from build123d import *

# Parameters (mm, degrees)
F0_W     = 30
F0_H     = 30
F1_DEPTH = 2
F3_DEPTH = 15
F4_W     = 8.5
F4_H     = 8.5
F5_DEPTH = 25
F6_W     = 2
F6_H     = 8
F7_DEPTH = 15
F8_W     = 5
F8_H     = 8
F9_DEPTH = 1


with BuildPart() as f1:
    # F0 (on Front) → F1 (new body)
    with BuildSketch(Plane.XZ):
        Rectangle(F0_W, F0_H)
    extrude(amount=F1_DEPTH)

    # F2 (on face) → F3 (join)
    with BuildSketch(Plane.XZ.offset(2)):
        Polygon((5.9, -11), (5.9, -13), (11.9, -13), (11.9, 0), (5.9, 0), (5.9, -2), (9.9, -2), (9.9, -11), align=None)
        Polygon((-9.9, -2), (-5.9, -2), (-5.9, 0), (-11.9, 0), (-11.9, -13), (-5.9, -13), (-5.9, -11), (-9.9, -11), align=None)
    extrude(amount=F3_DEPTH)

    # F4 (on face) → F5 (cut)
    with BuildSketch(Plane.XZ.offset(2)):
        with Locations((0, -1.25)):
            Rectangle(F4_W, F4_H)
    extrude(amount=-F5_DEPTH, mode=Mode.SUBTRACT)

    # F6 (on face) → F7 (join)
    with BuildSketch(Plane.XZ.offset(2)):
        with Locations((-7.263201, 9)):
            Rectangle(F6_W, F6_H)
        with Locations((7.263201, 9)):
            Rectangle(F6_W, F6_H)
    extrude(amount=F7_DEPTH)

    # F8 (on face) → F9 (cut)
    with BuildSketch(Plane.XZ.offset(2)):
        with Locations((0, 7)):
            Rectangle(F8_W, F8_H)
    extrude(amount=-F9_DEPTH, mode=Mode.SUBTRACT)


solid = f1.part
For this review, take the finished solid that the model builds, in its own axes (mm). A direction names the side the tool comes from. Round coordinates to 2 decimals unless told otherwise and drop trailing zeros. Order: outer loops, then holes, each group sorted by start corner. A loop starts at its lowest first (then second) coordinate and runs counter-clockwise, first axis right, second up. Notation, with made-up numbers: (43, 50.25) -> (78, 50.25) arc R20 cw to (78, 74.25) -> close; hole circle Ø1 at (38, -9). An arc over 180 degrees is marked (long way). Write item = value, one per line. Start each with the question number.
1) Tool access review of faces 1 (the face through (7, -9, 5)), 2 (the face through (8, -9, -2)), 3 (the face through (-5.9, -9, -1)), 4 (the face through (4.25, -1, -1)): name each direction out of +Z, -Z, +X, -X, +Y, -Y from which nothing blocks a thin tool from reaching the whole face with its end or side.
2) Take a section at C-C on y = -1.5. State the section outline as (x, z) points, plus the area to 3 significant figures.
3) The part is to be moulded in two halves that separate along Z. For faces 5 (the face through (9, -9, -13)), 6 (the face through (2.5, -1.5, 6.9)), 7 (the face through (-7, -17, 9)), say which applies: +Z half, -Z half, draft (parallel to the pull), parting line (faces both ways), or undercut.
4) Take a section at B-B on x = 2. State the section outline as (y, z) points.
5) Take a section at D-D on z = -7.75. State the section outline as (x, y) points.
6) Insertion check: pin 1 (1.2 mm diameter, centred on x = 7.5, y = -8, fed in from +Z); pin 2 (8 mm diameter, centred on y = -13.5, z = 8, fed in from +X); pin 3 (1.5 mm diameter, centred on y = -4.5, z = -2, fed in from +X). Each pin has a flat end and moves straight along its axis. Give the tip position at first contact, or say it passes through.
7) Take a section at A-A on y = -10.75. State the section outline as (x, z) points, plus the area to 3 significant figures.
8) To check wall thickness, follow line 1 (Z direction, x = -8, y = -5.25); line 2 (X direction, y = -11.75, z = -5.5); line 3 (Z direction, x = -8.75, y = -11.75). State the ranges of each line that lie inside material, in increasing order. Write a range as from..to.
Verdict:
q1.face_1 = +X, -X, -Y
q1.face_2 = -Y
q1.face_3 = +Z, -Z, -Y
q1.face_4 = +Y, -Y
q2.outline = (-15, -15) -> (15, -15) -> (15, 15) -> (-15, 15) -> close; hole (-4.25, -5.5) -> (4.25, -5.5) -> (4.25, 3) -> (2.5, 3) -> (2.5, 11) -> (-2.5, 11) -> (-2.5, 3) -> (-4.25, 3) -> close
q2.area = 788 mm2
q3.face_5 = -Z half
q3.face_6 = undercut
q3.face_7 = draft
q4.outline = (-2, -15) -> (0, -15) -> (0, -5.5) -> (-2, -5.5) -> close; (-2, 11) -> (-1, 11) -> (-1, 3) -> (0, 3) -> (0, 15) -> (-2, 15) -> close
q5.outline = (-15, -2) -> (-11.9, -2) -> (-11.9, -17) -> (-9.9, -17) -> (-9.9, -2) -> (9.9, -2) -> (9.9, -17) -> (11.9, -17) -> (11.9, -2) -> (15, -2) -> (15, 0) -> (-15, 0) -> close
q6.pin_1 = 13
q6.pin_2 = 8.26
q6.pin_3 = 11.9
q7.outline = (-11.9, -13) -> (-5.9, -13) -> (-5.9, -11) -> (-9.9, -11) -> (-9.9, -2) -> (-5.9, -2) -> (-5.9, 0) -> (-11.9, 0) -> close; (-8.26, 5) -> (-6.26, 5) -> (-6.26, 13) -> (-8.26, 13) -> close; (5.9, -13) -> (11.9, -13) -> (11.9, 0) -> (5.9, 0) -> (5.9, -2) -> (9.9, -2) -> (9.9, -11) -> (5.9, -11) -> close; (6.26, 5) -> (8.26, 5) -> (8.26, 13) -> (6.26, 13) -> close
q7.area = 116 mm2
q8.line_1 = -13..-11, -2..0, 5..13
q8.line_2 = -11.9..-9.9, 9.9..11.9
q8.line_3 = -13..-11, -2..0
